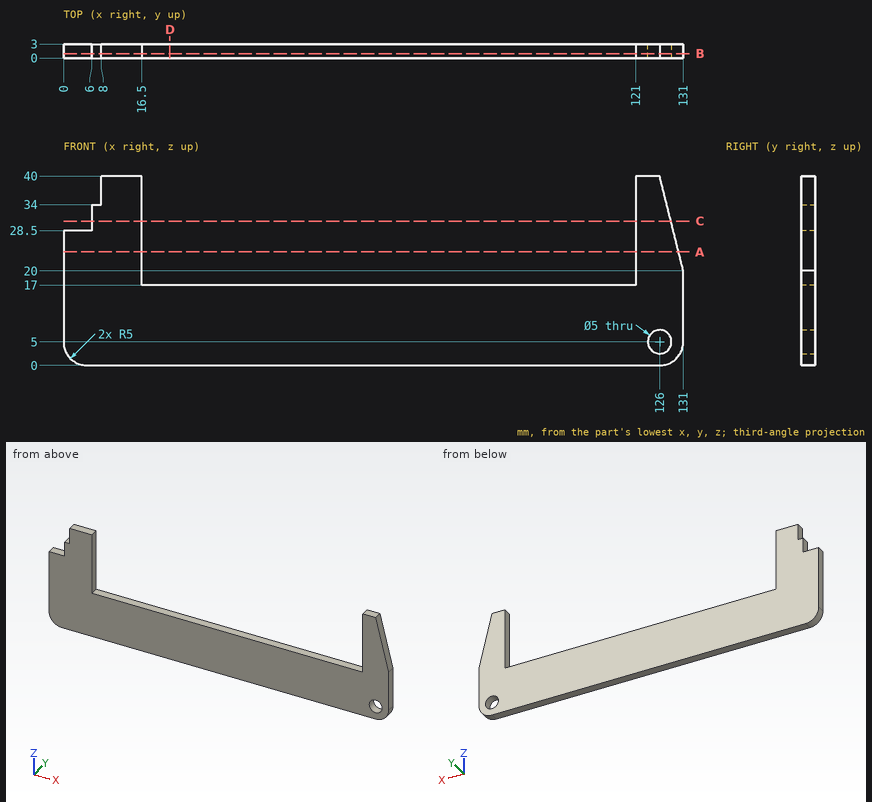
Part print with two shaded views. Sizes in mm from the minimum x, y, z corner. Round coordinates to 2 decimals unless told otherwise and drop trailing zeros. Order: outer loops, then holes, each group sorted by start corner. A loop starts at its lowest first (then second) coordinate and runs counter-clockwise, first axis right, second up. Notation, with made-up numbers: (56.5, 10.5) - (92.5, 10.5) arc R32 ccw to (92.5, 47.5) - close; hole circle Ø5 at (12.25, 78.25). An arc over 180 degrees is marked (long way). Answer in a Markdown table with one row per item. Add a question column.
(1) Probe L1, parallel to X at y = 1.8, z = 19.5; L2, parallel to X at y = 0.9, z = 21; L3, parallel to Z at x = 98, y = 2.8. List the from-to ranges inside material, lowest first. Write a range as [from, to].
(2) Band-saw the part on A-A on z = 24. List the corners of the cut face in (x, y), and give its area (3 significant figures).
(3) Band-saw the part on B-B on y = 0.95. List the corners of the cut face in (x, z).
(4) Drop flat-ended pins along their axis: pin 1 Ø1.5 at (y, z) = (1.5, 29) entering from +X; pin 2 Ø1.5 at (x, y) = (3.5, 1.5) entering from +Z; pin 3 Ø0.9 at (x, y) = (66, 1) entering from +Z. Give the stop position or say it passes through.
(5) Band-saw the part on C-C on z = 30.5. List the corners of the cut face in (x, y) (3 decimals).
(6) Band-saw the part on D-D on x = 22.5. List the corners of the cut face in (y, z).
Data:
| question | item | result |
|---|---|---|
| 1 | L1 | x = [0, 16.5], [121, 131] |
| 1 | L2 | x = [0, 16.5], [121, 130.75] |
| 1 | L3 | z = [0, 17] |
| 2 | outline | (0, 0) - (16.5, 0) - (16.5, 3) - (0, 3) - close; (121, 0) - (130, 0) - (130, 3) - (121, 3) - close |
| 2 | area | 76.5 mm^2 |
| 3 | outline | (0, 5) arc R5 ccw to (5, 0) - (126, 0) arc R5 ccw to (131, 5) - (131, 20) - (126, 40) - (121, 40) - (121, 17) - (16.5, 17) - (16.5, 40) - (8, 40) - (8, 34) - (6, 34) - (6, 28.5) - (0, 28.5) - close; hole circle Ø5 at (126, 5) |
| 4 | pin 1 | stops at x = 128.94 |
| 4 | pin 2 | stops at z = 28.5 |
| 4 | pin 3 | stops at z = 17 |
| 5 | outline | (6, 0) - (16.5, 0) - (16.5, 3) - (6, 3) - close; (121, 0) - (128.375, 0) - (128.375, 3) - (121, 3) - close |
| 6 | outline | (0, 0) - (3, 0) - (3, 17) - (0, 17) - close |
